CAD build for the part. Positions are in the model's coordinates, mm. A direction names the side the tool comes from. Round coordinates to 2 decimals unless told otherwise and drop trailing zeros. Loops run counter-clockwise (first coordinate to the right, second up) from the corner with the lowest first, then second, coordinate; pieces in that order, holes last.
from build123d import *

# Parameters (mm, degrees)
SKETCH6_W           = 25
SKETCH6_H           = 25
BOSS_EXTRUDE3_DEPTH = 4
SKETCH11_R          = 5
BOSS_EXTRUDE7_DEPTH = 15
SKETCH8_W           = 25
SKETCH8_H           = 12.5
BOSS_EXTRUDE5_DEPTH = 11
SKETCH12_R          = 2.25
CUT_EXTRUDE3_DEPTH  = 28.244265452
SKETCH9_W           = 1
SKETCH9_H           = 7
CUT_EXTRUDE2_DEPTH  = 11
CUT_EXTRUDE4_DEPTH  = 1.5
FILLET2_R           = 5


with BuildPart() as part:
    # Sketch6 → Boss-Extrude3 (new body)
    with BuildSketch(Plane.XZ):
        Rectangle(SKETCH6_W, SKETCH6_H)
    extrude(amount=BOSS_EXTRUDE3_DEPTH)

    # Sketch11 → Boss-Extrude7 (add)
    with BuildSketch(Plane(origin=(0, 0, 0), x_dir=(1, 0, 0), z_dir=(0, 1, 0))):
        with Locations(Location((-14, 0, 0), (0, 0, 270))):
            Circle(SKETCH11_R)
        with Locations(Location((14, 0, 0), (0, 0, 270))):
            Circle(SKETCH11_R)
    extrude(amount=-BOSS_EXTRUDE7_DEPTH)

    # Sketch8 → Boss-Extrude5 (add)
    with BuildSketch(Plane.XZ.offset(4)):
        with Locations((0, -6.25)):
            Rectangle(SKETCH8_W, SKETCH8_H)
    extrude(amount=BOSS_EXTRUDE5_DEPTH)

    # Sketch12 → Cut-Extrude3 (cut, through all)
    with BuildSketch(Plane(origin=(0, 0, 0), x_dir=(1, 0, 0), z_dir=(0, 1, 0))):
        with Locations(Location((-14, 0, 0), (0, 0, 270))):
            Circle(SKETCH12_R)
        with Locations(Location((14, 0, 0), (0, 0, 270))):
            Circle(SKETCH12_R)
    extrude(amount=-CUT_EXTRUDE3_DEPTH, mode=Mode.SUBTRACT)

    # Sketch9 → Cut-Extrude2 (cut)
    with BuildSketch(Plane.XZ.offset(15)):
        with Locations((0, -3.5)):
            Rectangle(SKETCH9_W, SKETCH9_H)
    extrude(amount=-CUT_EXTRUDE2_DEPTH, mode=Mode.SUBTRACT)

    # Sketch13 → Cut-Extrude4 (cut)
    with BuildSketch(Plane.XZ.offset(4)):
        with BuildLine():
            Line((-11, 0), (-11, 12.5))
            Line((-11, 12.5), (11, 12.5))
            Line((11, 12.5), (11, 0))
            ThreePointArc((11, 0), (0, -11), (-11, 0))
        make_face()
    extrude(amount=CUT_EXTRUDE4_DEPTH, mode=Mode.SUBTRACT)

    # Fillet2
    fillet2_edges = [part.edges().sort_by_distance(p)[0] for p in [
        (-12.5, -7.5, -4.769696007),
        (12.5, -7.5, -4.769696007),
        (-12.5, -2, 12.5),
        (12.5, -2, 12.5),
    ]]
    fillet(fillet2_edges, radius=FILLET2_R)


solid = part.part
Item 1: Wall check: L1, parallel to Y at x = -6, z = -6.75; L2, parallel to X at y = -7, z = -0.75; L3, parallel to X at y = -3, z = 0. Give the ranges that are in metal, low to high.
Verdict:
L1: y = -15 to -5.5, -4 to 0
L2: x = -18.94 to -16.12, -11.88 to -0.5, 0.5 to 11.88, 16.12 to 18.94
L3: x = -19 to -16.25, -11.75 to 11.75, 16.25 to 19
Item 2: Cut at B-B (x = -13). List the corners of the cut face in (y, z), plus the area to 3 significant figures.
Verdict:
outline: (-15, -7.19) - (0, -7.19) - (0, -2.02) - (-15, -2.02) - close; (-15, 2.02) - (0, 2.02) - (0, 4.9) - (-15, 4.9) - close
area: 121 mm2
Item 3: 3-axis set-ups, long thin cutter, end or side, ignore diameter. For faces 4 (the flat face through (-12.5, -7, -11)), 5 (the cylindrical face through (0, -5, -11)), 6 (the flat face through (0, -10, -7)): which of +Z, -Z, +X, -X, +Y, -Y reach the whole face in a straight line?
Verdict:
face 4: -Z, -X, +Y, -Y
face 5: +Z
face 6: +Z, -Y
Item 4: Mould opens along Z. For faces 1 (the flat face through (-11, -5, 2)), 2 (the flat face through (-5, -10, 0)), 3 (the cylindrical face through (11.804, -7.395, -0.488)) say: released by +Z, released by -Z, zero draft, split by the parting line, or undercut.
Verdict:
face 1: zero draft
face 2: released by +Z
face 3: undercut
Item 5: Cut at D-D (x = 0). List the corners of the cut face in (y, z).
Verdict:
outline: (-15, -12.5) - (0, -12.5) - (0, 12.5) - (-4, 12.5) - (-4, -11) - (-5.5, -11) - (-5.5, -7) - (-15, -7) - close
Item 6: Flat gauge pins, fed straight in: P1, Ø0.8, axis at x = 0, y = -9.5, coming from the +Z side; P2, Ø5, axis at x = 5, z = 2.5, coming from the +Y side; P3, Ø4, axis at x = -6, y = -12.5, coming from the +Z side; P4, Ø0.8, axis at y = -4.5, z = 2.5, coming from the -X side. Where does each tip first touch, or does it go through?
Verdict:
P1: stops at z = -7
P2: stops at y = 0
P3: stops at z = 0
P4: stops at x = -18.54
Item 7: Cut at C-C (z = 3). List the corners of the cut face in (x, y), plus the area to 3 significant figures.
Verdict:
outline: (-18, -15) - (-10, -15) - (-10, -5.5) - (-11, -5.5) - (-11, -4) - (11, -4) - (11, -5.5) - (10, -5.5) - (10, -15) - (18, -15) - (18, 0) - (-18, 0) - close
area: 317 mm2
Item 8: Cut at A-A (y = -7). List the corners of the cut face in (x, z).
Verdict:
outline: (-15.75, -4.68) arc R5 cw to (-12.5, -9.37) - (-12.5, -12.5) - (12.5, -12.5) - (12.5, -9.37) arc R5 cw to (15.75, -4.68) arc R5 ccw (long way) to (9, 0) - (0.5, 0) - (0.5, -7) - (-0.5, -7) - (-0.5, 0) - (-9, 0) arc R5 ccw (long way) to start; hole circle Ø4.5 at (-14, 0); hole circle Ø4.5 at (14, 0)
